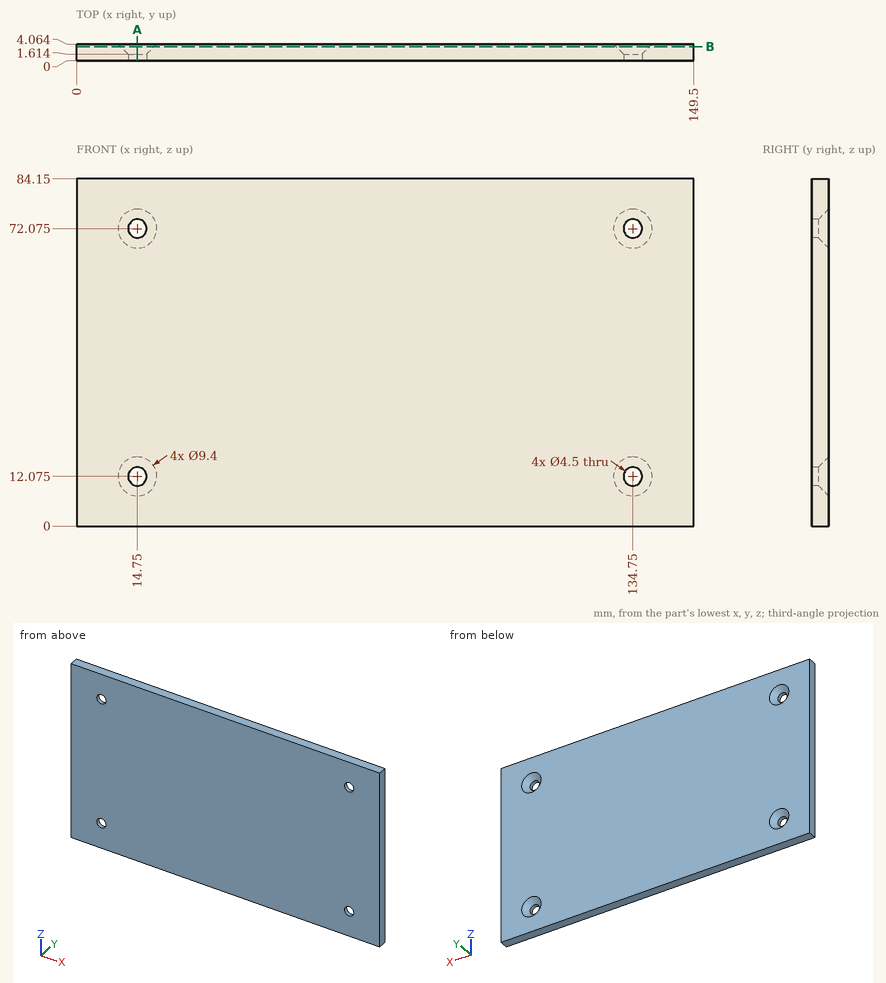
Check sheet for the drawn part. Datum: minimum x, y, z corner. Units: mm. Round coordinates to 2 decimals unless told otherwise and drop trailing zeros. Loops run counter-clockwise (first coordinate to the right, second up) from the corner with the lowest first, then second, coordinate; pieces in that order, holes last. Notation, with made-up numbers: (-37.5, 66) -> (-4.5, 66) arc R32 cw to (-4.5, 103) -> close; hole circle Ø10 at (47.25, 18). An arc over 180 degrees is marked (long way). Put each result on its own line as item: value. Start each with the question number.
1. Gauge pin test, flat ends, axial feed: pin 1 (3 mm diameter, centred on x = 15, z = 67.5, fed in from +Y); pin 2 (5 mm diameter, centred on x = 14.75, z = 72.075, fed in from +Y); pin 3 (2.5 mm diameter, centred on x = 14.75, z = 12.075, fed in from +Y). Record the tip position at first contact, or that the pin passes through.
2. Section check B-B (y = 3.4). Enter the section's corners in (x, z) (3 decimals).
3. Section check A-A (x = 14.75). Enter the section's corners in (y, z) (3 decimals), plus the area to 3 significant figures.
4. Scan lines: probe 1 along Z at (x, y) = (14.75, 0.7) (3 decimals); probe 2 along X at (y, z) = (2.85, 74); probe 3 along X at (y, z) = (2.8, 9). Record each from-to range of solid material in increasing order.
Findings:
1. pin 1: stops at y = 4.06
1. pin 2: stops at y = 1.86
1. pin 3: passes through
2. outline: (0, 0) -> (149.5, 0) -> (149.5, 84.15) -> (0, 84.15) -> close; hole circle Ø8.072 at (14.75, 12.075); hole circle Ø8.072 at (14.75, 72.075); hole circle Ø8.072 at (134.75, 12.075); hole circle Ø8.072 at (134.75, 72.075)
3. outline: (0, 0) -> (4.064, 0) -> (4.064, 7.375) -> (1.614, 9.825) -> (0, 9.825) -> close; (0, 14.325) -> (1.614, 14.325) -> (4.064, 16.775) -> (4.064, 67.375) -> (1.614, 69.825) -> (0, 69.825) -> close; (0, 74.325) -> (1.614, 74.325) -> (4.064, 76.775) -> (4.064, 84.15) -> (0, 84.15) -> close
3. area: 293 mm^2
4. probe 1: z = 0 to 9.825, 14.325 to 69.825, 74.325 to 84.15
4. probe 2: x = 0 to 11.84, 17.66 to 131.84, 137.66 to 149.5
4. probe 3: x = 0 to 13.22, 16.28 to 133.22, 136.28 to 149.5
